Input: dimensioned drawing with shaded views. Units: mm. Origin: part minimum x, y, z. Round coordinates to 2 decimals unless told otherwise and drop trailing zeros. Loops run counter-clockwise (first coordinate to the right, second up) from the corner with the lowest first, then second, coordinate; pieces in that order, holes last. Notation, with made-up numbers: M 85.25,83.25 L 113.25,83.25 A19 cw 113.25,92.25 Z; hole C 66,4 d1. An arc over 180 degrees is marked long. One line per item, written item: value.
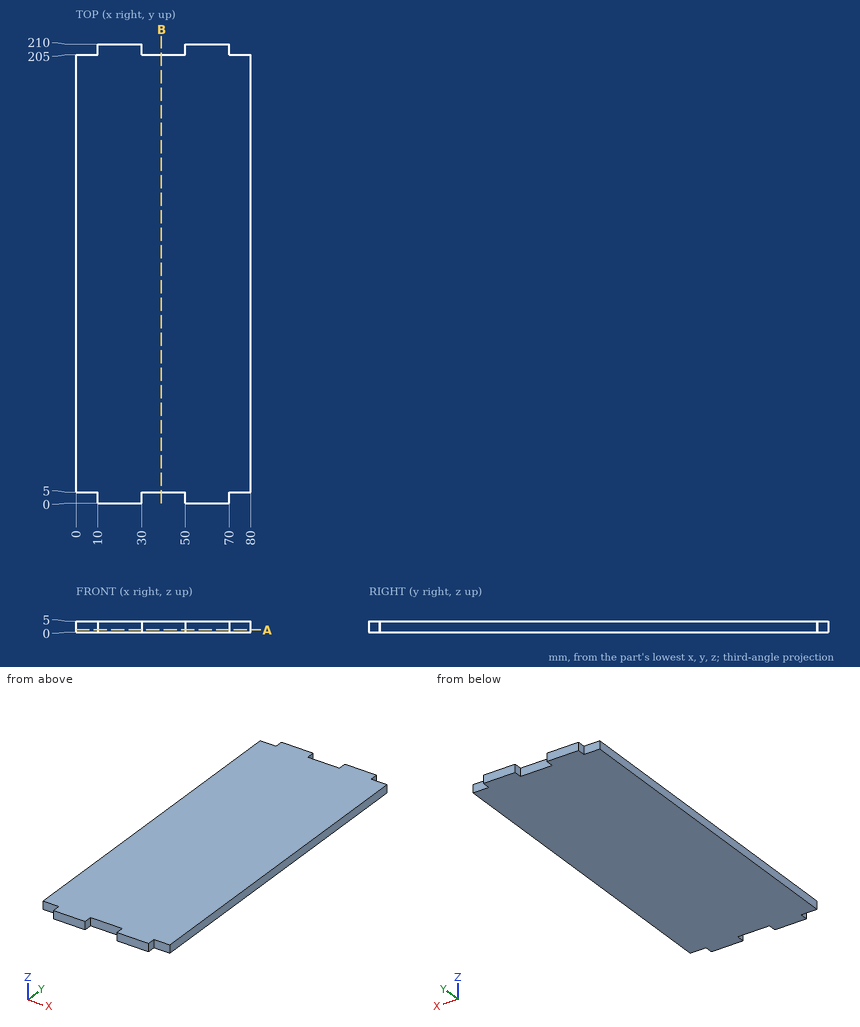
1. Pin query (flat end, axial travel): pin 1 (1.5 mm diameter, centred on y = 3, z = 3, fed in from -X); pin 2 (1.5 mm diameter, centred on y = 207.5, z = 3, fed in from +X); pin 3 (1.5 mm diameter, centred on x = 73.5, z = 2, fed in from -Y). Return the tip coordinate at first contact, or that it passes through.
Report:
pin 1: stops at x = 10
pin 2: stops at x = 70
pin 3: stops at y = 5
2. Section query A-A (z = 1). Return the cut outline in (x, y).
Report:
outline: M 0,5 L 10,5 L 10,0 L 30,0 L 30,5 L 50,5 L 50,0 L 70,0 L 70,5 L 80,5 L 80,205 L 70,205 L 70,210 L 50,210 L 50,205 L 30,205 L 30,210 L 10,210 L 10,205 L 0,205 Z
3. Ray query, line 1 (Y direction, x = 46, z = 1.5). Return the intervals inside material, ascending. Write a range as [from, to].
Report:
line 1: y = [5, 205]
4. Section query B-B (x = 39). Return the cut outline in (y, z), and give its area (3 significant figures).
Report:
outline: M 5,0 L 205,0 L 205,5 L 5,5 Z
area: 1,000 mm2
